```python
from build123d import *

# Parameters (mm, degrees)
BOSS_EXTRUDE1_DEPTH = 47.625
SKETCH2_R           = 3.175
CUT_EXTRUDE1_DEPTH  = 98.205482527


with BuildPart() as part:
    # Sketch1 → Boss-Extrude1 (new, symmetric)
    with BuildSketch(Plane(origin=(0, 0, 0), x_dir=(1, 0, 0), z_dir=(0, 1, 0))):
        Polygon((-14.664696837, 0), (-7.332348419, -12.7), (7.332348419, -12.7), (14.664696837, 0), (7.332348419, 12.7), (-7.332348419, 12.7), align=None)
    extrude(amount=BOSS_EXTRUDE1_DEPTH, both=True)

    # Sketch2 → Cut-Extrude1 (cut, through all)
    with BuildSketch(Plane(origin=(0, 47.625, 0), x_dir=(1, 0, 0), z_dir=(0, 1, 0))):
        with Locations(Location((0, 0, 0), (0, 0, 270))):
            Circle(SKETCH2_R)
    extrude(amount=-CUT_EXTRUDE1_DEPTH, mode=Mode.SUBTRACT)


solid = part.part
```
Geometry check sheet. Reference: the model listing, model coordinates, mm. Give positions to 0.01 mm unless a question says otherwise; leave off trailing zeros. Write each loop counter-clockwise with the first axis right and the second up, starting at its lowest first coordinate (ties: lowest second). Pieces come first, ordered by that corner, then holes.
1) Section check B-B, the plane y = 17. Record the boundary of the cut face in (x, z) (3 decimals).
2) Material ranges on L1, parallel to X at y = 14.5, z = 0 (3 decimals); L2, parallel to Z at x = 13.5, y = 3; L3, parallel to X at y = -43.5, z = -9.75, recorded low to high.
3) Release check for a two-part mould opening along Z. For faces 1 (the cylindrical face through (-1.93, 0.67, -2.52)), 2 (the flat face through (11.05, 0.67, -6.26)), 3 (the flat face through (3, 47.625, -3)) record: pulls with the +Z half, pulls with the -Z half, needs draft (parallel to the pull), parting line crosses it, or undercut.
4) Section check A-A, the plane x = 0. Record the boundary of the cut face in (y, z) (3 decimals).
5) Section check D-D, the plane x = -10. Record the boundary of the cut face in (y, z) (1 decimal), and give its area (3 significant figures).
6) Section check C-C, the plane z = -1.25. Record the boundary of the cut face in (x, y) (3 decimals), and give its area (3 significant figures).
Computed:
1. outline: (-14.665, 0) - (-7.332, -12.7) - (7.332, -12.7) - (14.665, 0) - (7.332, 12.7) - (-7.332, 12.7) - close; hole circle Ø6.35 at (0, 0)
2. L1: x = -14.665 to -3.175, 3.175 to 14.665
2. L2: z = -2.02 to 2.02
2. L3: x = -9.04 to 9.04
3. face 1: undercut
3. face 2: pulls with the -Z half
3. face 3: needs draft
4. outline: (-47.625, -12.7) - (47.625, -12.7) - (47.625, -3.175) - (-47.625, -3.175) - close; (-47.625, 3.175) - (47.625, 3.175) - (47.625, 12.7) - (-47.625, 12.7) - close
5. outline: (-47.6, -8.1) - (47.6, -8.1) - (47.6, 8.1) - (-47.6, 8.1) - close
5. area: 1,540 mm2
6. outline: (-13.943, -47.625) - (-2.919, -47.625) - (-2.919, 47.625) - (-13.943, 47.625) - close; (2.919, -47.625) - (13.943, -47.625) - (13.943, 47.625) - (2.919, 47.625) - close
6. area: 2,100 mm2
